Build history of the part. All positions in model axes, mm. Face numbers are marked on the shaded views. A direction names the side the tool comes from. Round coordinates to 2 decimals unless told otherwise and drop trailing zeros. Loops run counter-clockwise (first coordinate to the right, second up) from the corner with the lowest first, then second, coordinate; pieces in that order, holes last. Notation, with made-up numbers: M -25.75,65.5 L 28.25,65.5 A27 ccw 28.25,92.5 Z; hole C 41,5.5 d11. An arc over 180 degrees is marked long. One line per item, written item: value.
```python
from build123d import *

# Parameters (mm, degrees)
F1_DEPTH = 63.5
F0_W     = 25.4
F0_H     = 19.05
F2_DEPTH = 25.4
F4_DEPTH = 7.9375
F5_R     = 5.08


with BuildPart() as f1:
    # F0 (on Front) → F1 (new body, symmetric)
    with BuildSketch(Plane.XZ):
        Polygon((41.275, -9.525), (41.275, 9.525), (22.225, 9.525), (-41.275, 9.525), (-41.275, -9.525), align=None)
    extrude(amount=F1_DEPTH, both=True)

    # F0 (on Front) → F2 (join, symmetric)
    with BuildSketch(Plane.XZ):
        with BuildLine():
            Line((22.225, 9.525), (41.275, 9.525))
            Line((41.275, 9.525), (41.275, 27.0002))
            ThreePointArc((41.275, 27.0002), (45.9246798487, 38.2255201513), (57.15, 42.8752))
            Line((57.15, 42.8752), (60.325, 42.8752))
            Line((60.325, 42.8752), (60.325, 61.9252))
            Line((60.325, 61.9252), (57.15, 61.9252))
            ThreePointArc((57.15, 61.9252), (32.4542956671, 51.6959043329), (22.225, 27.0002))
            Line((22.225, 27.0002), (22.225, 9.525))
        make_face()
        with Locations((73.025, 52.4002)):
            Rectangle(F0_W, F0_H)
    extrude(amount=F2_DEPTH, both=True)

    # F0 (on Front) → F3 (revolve)
    with BuildSketch(Plane.XZ):
        Polygon((85.725, 61.9252), (85.725, 42.8752), (85.725, 38.1), (111.125, 38.1), (111.125, 66.675), (85.725, 66.675), align=None)
    revolve(axis=Axis((85.725, 0, 52.3875), (0, 0, 1)))

    # F0 (on Front) → F4 (join, symmetric)
    with BuildSketch(Plane.XZ):
        with BuildLine():
            Line((-41.275, 9.525), (22.225, 9.525))
            Line((22.225, 9.525), (22.225, 27.0002))
            ThreePointArc((22.225, 27.0002), (32.4542956671, 51.6959043329), (57.15, 61.9252))
            add(Edge.make_bspline(
                [(57.15, 61.9252), (24.6527968383, 61.9252), (-30.2506246056, 64.332675823), (-39.2470384075, 24.7092637795), (-41.275, 9.525)],
                knots=[0, 0, 0, 0, 0.5726218411, 1, 1, 1, 1], degree=3))
        make_face()
    extrude(amount=F4_DEPTH, both=True)

    # F5
    f5_edges = [f1.edges().sort_by_distance(p)[0] for p in [
        (-41.275, -63.5, 0),
        (41.275, -63.5, 0),
        (41.275, 63.5, 0),
        (-41.275, 63.5, 0),
    ]]
    fillet(f5_edges, radius=F5_R)


solid = f1.part
```
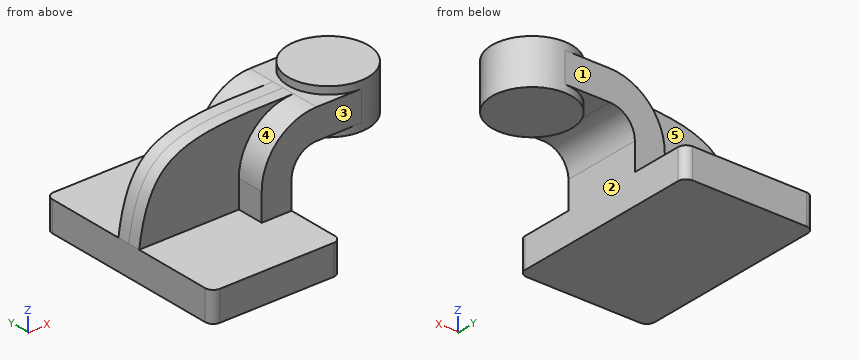
Item 1: Drop flat-ended pins along their axis: P1, Ø3, axis at x = -21.5, z = 48.5, coming from the +Y side; P2, Ø10, axis at x = -9.5, y = -33, coming from the +Z side (3 decimals); P3, Ø5, axis at x = 50.5, z = 40, coming from the +Y side; P4, Ø4, axis at x = 72, y = 29, coming from the +Z side. Give the stop position or say it passes through.
Check values:
P1: stops at y = 7.94
P2: stops at z = 9.525
P3: stops at y = 25.4
P4: passes through
Item 2: Which spindle directions (+Z, -Z, +X, -X, +Y, -Y) get a long thin tool onto all of the face, cutting with end or side? Do the marked faces 1, 2, 3, 4 and 5. Say none if no direction does.
Check values:
face 1: +Z, +X, -X, +Y
face 2: -Z, +X, +Y, -Y
face 3: +Z, +X, -X, -Y
face 4: +Z, -X, -Y
face 5: +Z, -X, +Y
Item 3: Slice it at B-B, the plane y = -19. Give the cut face in (x, z) (3 decimals).
Check values:
outline: M -41.275,-9.525 L 41.275,-9.525 L 41.275,27 A15.875 cw 57.15,42.875 L 68.868,42.875 L 68.868,38.1 L 102.582,38.1 L 102.582,66.675 L 68.868,66.675 L 68.868,61.925 L 57.15,61.925 A34.925 ccw 22.225,27 L 22.225,9.525 L -41.275,9.525 Z
Item 4: Slice it at A-A, the plane z = 3. Give the cut face in (x, y) (3 decimals).
Check values:
outline: M -41.275,-58.42 A5.08 ccw -36.195,-63.5 L 36.195,-63.5 A5.08 ccw 41.275,-58.42 L 41.275,58.42 A5.08 ccw 36.195,63.5 L -36.195,63.5 A5.08 ccw -41.275,58.42 Z
Item 5: Wall check: line 1 along Z through (x, y) = (0, -29) (3 decimals); line 2 along X through (y, z) = (-13, 12) (3 decimals); line 3 along Y through (x, z) = (24.5, 12). Give the ranges that are in metal, low to high.
Check values:
line 1: z = -9.525 to 9.525
line 2: x = 22.225 to 41.275
line 3: y = -25.4 to 25.4
